from build123d import *

# Parameters (mm, degrees)
SKETCH1_R               = 7
SKETCH1_R_2             = 4
BOSS_EXTRUDE1_DEPTH     = 7
CUT_EXTRUDE1_REACH      = 14.124
CUT_EXTRUDE1_END_RADIUS = 7
SKETCH2_R               = 1.75
CHAMFER1_SIZE           = 0.5


with BuildPart() as part:
    # Sketch1 → Boss-Extrude1 (new body)
    with BuildSketch(Plane(origin=(0, 0, 0), x_dir=(1, 0, 0), z_dir=(0, 1, 0))):
        with Locations(Location((0, 0, 0), (0, 0, 270))):
            Circle(SKETCH1_R)
        with Locations(Location((0, 0, 0), (0, 0, 270))):
            Circle(SKETCH1_R_2, mode=Mode.SUBTRACT)
    extrude(amount=BOSS_EXTRUDE1_DEPTH)

    # Cut-Extrude1: up to this cylinder (the profile starts inside it)
    cut_extrude1_end = Plane(origin=(0, 3.5, 0), z_dir=(0, -1, 0)) * Cylinder(CUT_EXTRUDE1_END_RADIUS, 43.248, mode=Mode.PRIVATE)
    # Sketch2 → Cut-Extrude1 (cut, up to the surface)
    with BuildSketch(Plane.XY, mode=Mode.PRIVATE) as cut_extrude1_sk1:
        with Locations((0, 3.5)):
            Circle(SKETCH2_R)
    cut_extrude1_tool1 = extrude(cut_extrude1_sk1.sketch, amount=-CUT_EXTRUDE1_REACH, mode=Mode.PRIVATE) & cut_extrude1_end
    add(cut_extrude1_tool1.solids().sort_by_distance((0, 3.5, 0))[0], mode=Mode.SUBTRACT)

    # Chamfer1
    chamfer1_edges = [part.edges().sort_by_distance(p)[0] for p in [
        (0, 0, -7),
        (0, 7, -7),
        (0, 0, -4),
        (0, 7, -4),
    ]]
    chamfer(chamfer1_edges, length=CHAMFER1_SIZE)


solid = part.part
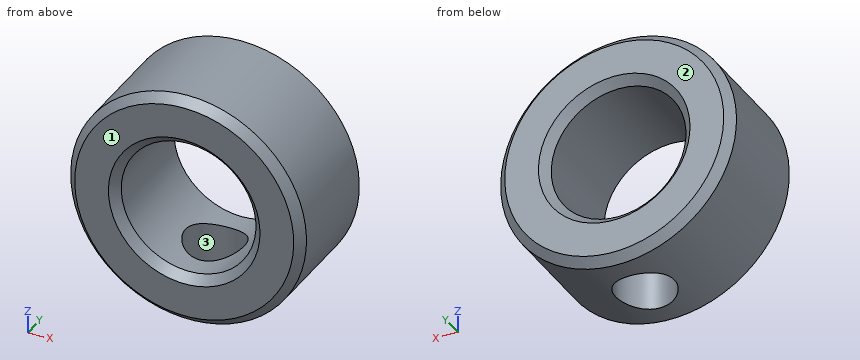
The listing builds one solid part. Answer for the finished solid, in the listing's coordinates (mm). Face numbers are marked on the shaded views. Give positions to 0.01 mm unless a question says otherwise; leave off trailing zeros. Order: outer loops, then holes, each group sorted by start corner. A loop starts at its lowest first (then second) coordinate and runs counter-clockwise, first axis right, second up. Notation, with made-up numbers: (5, 43.5) - (29, 43.5) arc R22 ccw to (29, 55.5) - close; hole circle Ø6 at (87.5, -19). An arc over 180 degrees is marked (long way). Use one line per item in the form item = value.
1) Consider probe 1 along X at (y, z) = (2.75, 0); probe 2 along Z at (x, y) = (-1, 1.75); probe 3 along Z at (x, y) = (-2, 5.25). Determine where each line is inside the solid, lowest interval first. Write a range as [from, to].
Verdict:
probe_1 = [-7, -4], [4, 7]
probe_2 = [-6.93, -3.87], [3.87, 6.93]
probe_3 = [-6.71, -3.46], [3.46, 6.71]
2) Find section A-A on z = 0. Determine the outline of the cut face in (x, y).
Verdict:
outline = (-7, 0.5) - (-6.5, 0) - (-4.5, 0) - (-4, 0.5) - (-4, 6.5) - (-4.5, 7) - (-6.5, 7) - (-7, 6.5) - close; (4, 0.5) - (4.5, 0) - (6.5, 0) - (7, 0.5) - (7, 6.5) - (6.5, 7) - (4.5, 7) - (4, 6.5) - close
3) Find section C-C on y = 6.75. Determine the outline of the cut face in (x, z).
Verdict:
outline = circle Ø13.5 at (0, 0); hole circle Ø8.5 at (0, 0)
4) Each of these flat-tipped pins is pushed along its axis until it touches: pin 1 (3 mm diameter, centred on x = 4.5, y = 1.5, fed in from +Z); pin 2 (1 mm diameter, centred on x = -4.5, y = 2.5, fed in from -Z). Where does it stop, or does it pass through?
Verdict:
pin_1 = 6.32
pin_2 = -5.74
5) The mould has two halves that part along Y. Classify the marked faces 1, 2 and 3: released by +Y, released by -Y, zero draft, split by the parting line, or undercut.
Verdict:
face_1 = released by -Y
face_2 = released by +Y
face_3 = undercut
6) Find section B-B on x = 0. Determine the outline of the cut face in (y, z).
Verdict:
outline = (0, -6.5) - (0.5, -7) - (1.75, -7) - (1.75, -4) - (0.5, -4) - (0, -4.5) - close; (0, 4.5) - (0.5, 4) - (6.5, 4) - (7, 4.5) - (7, 6.5) - (6.5, 7) - (0.5, 7) - (0, 6.5) - close; (5.25, -7) - (6.5, -7) - (7, -6.5) - (7, -4.5) - (6.5, -4) - (5.25, -4) - close
7) Find section D-D on y = 2.5. Determine the outline of the cut face in (x, z), and give its area (3 significant figures).
Verdict:
outline = (-1.44, -6.85) - (-1.44, -3.73) arc R4 cw (long way) to (1.44, -3.73) - (1.44, -6.85) arc R7 ccw (long way) to start
area = 94.9 mm^2
